```python
from build123d import *

# Parameters (mm, degrees)
SKETCH1_R           = 2.5
BOSS_EXTRUDE1_DEPTH = 3


with BuildPart() as part:
    # Sketch1 → Boss-Extrude1 (new body)
    with BuildSketch(Plane.XY):
        with BuildLine():
            Line((34.37, 75.95596391), (-15.63, 75.95596391))
            Line((-15.63, 75.95596391), (-15.63, 78.95596391))
            Line((-15.63, 78.95596391), (-41.63, 78.95596391))
            Line((-41.63, 78.95596391), (-41.63, 75.95596391))
            Line((-41.63, 75.95596391), (-60.44, 75.95596391))
            Line((-60.44, 75.95596391), (-60.44, 43.95596391))
            Line((-60.44, 43.95596391), (-63.44, 43.95596391))
            Line((-63.44, 43.95596391), (-63.44, 3.95596391))
            Line((-63.44, 3.95596391), (-60.44, 3.95596391))
            Line((-60.44, 3.95596391), (-60.44, -36.04403609))
            Line((-60.44, -36.04403609), (-63.44, -36.04403609))
            Line((-63.44, -36.04403609), (-63.44, -76.04403609))
            Line((-63.44, -76.04403609), (-60.44, -76.04403609))
            Line((-60.44, -76.04403609), (-15.324347337, -76.04403609))
            Line((-15.324347337, -76.04403609), (-15.324347337, -36.04403609))
            ThreePointArc((-15.324347337, -36.04403609), (0.56, -20.159688753), (16.444347337, -36.04403609))
            Line((16.444347337, -36.04403609), (16.444347337, -76.04403609))
            Line((16.444347337, -76.04403609), (60.37, -76.04403609))
            Line((60.37, -76.04403609), (60.37, 75.95596391))
            Line((60.37, 75.95596391), (60.37, 78.95596391))
            Line((60.37, 78.95596391), (34.37, 78.95596391))
            Line((34.37, 78.95596391), (34.37, 75.95596391))
        make_face()
        with Locations((-40.44, -66.04403609)):
            Circle(SKETCH1_R, mode=Mode.SUBTRACT)
        with Locations((40.37, -66.04403609)):
            Circle(SKETCH1_R, mode=Mode.SUBTRACT)
    extrude(amount=BOSS_EXTRUDE1_DEPTH)


solid = part.part
```
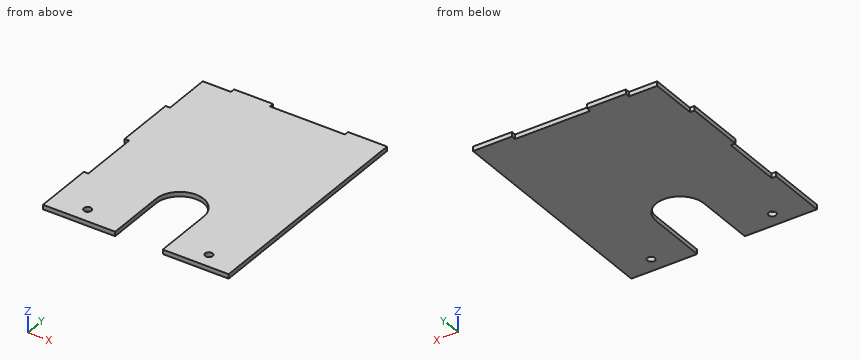
Input: part model. Units: mm. Frame: model coordinates. Coordinates: 2 decimals unless noted, no trailing zeros. Write each loop counter-clockwise with the first axis right and the second up, starting at its lowest first coordinate (ties: lowest second). Pieces come first, ordered by that corner, then holes. Notation, with made-up numbers: (67, 24.25) - (113, 24.25) arc R18 ccw to (113, 28.25) - close; hole circle Ø8 at (74, 27). An arc over 180 degrees is marked (long way). Put each result on its own line as item: value. Start each with the question number.
1) Contact query for flat-ended pins moving along their axis: pin 1 (0.9 mm diameter, centred on y = -17.5, z = 1, fed in from -X); pin 2 (1.5 mm diameter, centred on y = 78, z = 1.5, fed in from -X); pin 3 (4.5 mm diameter, centred on x = -40.44, y = -66.04, fed in from +Z); pin 4 (1.5 mm diameter, centred on x = -62.5, z = 1.5, fed in from +Y). Output: stop coordinate, or through.
2) Cut plane C-C (x = 0.56). Return the cut outline in (y, z).
3) Cut plane A-A (y = -55). Return the cut outline in (x, z).
4) Cut plane D-D (y = -29). Return the cut outline in (x, z).
5) Ray query, L1, parallel to Y at x = -40.44, z = 1.9; L2, parallel to X at y = -53, z = 2.1; L3, parallel to X at y = 50, z = 1.15. Return the intervals inside material, ascending.
6) Cut plane B-B (z = 2). Return the cut outline in (x, y), plus the area to 3 significant figures.
Resolved:
1. pin 1: stops at x = -60.44
1. pin 2: stops at x = -41.63
1. pin 3: passes through
1. pin 4: stops at y = 43.96
2. outline: (-20.16, 0) - (75.96, 0) - (75.96, 3) - (-20.16, 3) - close
3. outline: (-63.44, 0) - (-15.32, 0) - (-15.32, 3) - (-63.44, 3) - close; (16.44, 0) - (60.37, 0) - (60.37, 3) - (16.44, 3) - close
4. outline: (-60.44, 0) - (-13.68, 0) - (-13.68, 3) - (-60.44, 3) - close; (14.8, 0) - (60.37, 0) - (60.37, 3) - (14.8, 3) - close
5. L1: y = -76.04 to -68.54, -63.54 to 78.96
5. L2: x = -63.44 to -15.32, 16.44 to 60.37
5. L3: x = -60.44 to 60.37
6. outline: (-63.44, -76.04) - (-15.32, -76.04) - (-15.32, -36.04) arc R15.88 cw to (16.44, -36.04) - (16.44, -76.04) - (60.37, -76.04) - (60.37, 78.96) - (34.37, 78.96) - (34.37, 75.96) - (-15.63, 75.96) - (-15.63, 78.96) - (-41.63, 78.96) - (-41.63, 75.96) - (-60.44, 75.96) - (-60.44, 43.96) - (-63.44, 43.96) - (-63.44, 3.96) - (-60.44, 3.96) - (-60.44, -36.04) - (-63.44, -36.04) - close; hole circle Ø5 at (-40.44, -66.04); hole circle Ø5 at (40.37, -66.04)
6. area: 17,100 mm2
